CAD build for the part. Positions are in the model's coordinates, mm. Coordinates: 2 decimals unless noted, no trailing zeros. Loops run counter-clockwise (first coordinate to the right, second up) from the corner with the lowest first, then second, coordinate; pieces in that order, holes last. Notation, with made-up numbers: (-17.5, 56) -> (-9.5, 56) arc R3 ccw to (-9.5, 60) -> close; hole circle Ø5 at (24, 41.5). An arc over 180 degrees is marked (long way). Return JSON: item names as keys, results as strings. Group by question number.
(1) Probe L1, parallel to X at y = -20, z = 2.05 (3 decimals); L2, parallel to Y at x = -24.5, z = 1.05; L3, parallel to X at y = -9, z = 2.2 (3 decimals). List the from-to ranges inside material, lowest first.
(2) Flat gauge pin, fed straight in: pin 1 Ø12 at (x, y) = (-93.5, -21) entering from +Z. Where does the tip first touch, or does it go through?
(3) Saw through at C-C on z = 0.8. Give the number of separate pieces and of enclosed holes in the cut face, then the cut area to 3 significant figures.
(4) Saw through at B-B on y = -54.5. Write the cut outline in (x, z) (3 decimals).
(5) Saw through at A-A on x = -134.5. Write the cut outline in (y, z), then the cut area to 3 significant figures.
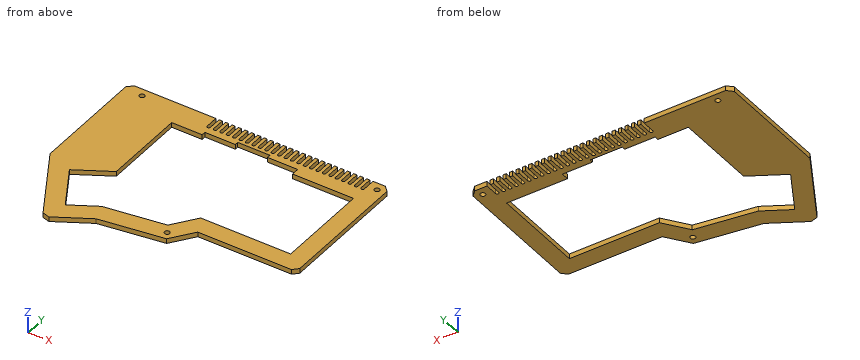
```python
from build123d import *

# Parameters (mm, degrees)
ESQUISSE1_R             = 1.6
BOSS_EXTRU_1_DEPTH      = 3
ENL_V_MAT_EXTRU_1_DEPTH = 10


with BuildPart() as part:
    # Esquisse1 → Boss.-Extru.1 (new body)
    with BuildSketch(Plane.XY):
        Polygon((5.525007543, 0.072428093), (2.276763789, 3.320852512), (-154.236345188, 3.320852512), (-157.478985875, 0.078211825), (-157.478985875, -70.04068474), (-131.779420125, -114.771472067), (-127.355917516, -115.9649154), (-106.081983802, -103.720194839), (-66.092540926, -97.775797545), (-55.98795635, -83.933633781), (2.418252352, -83.933633781), (5.525007543, -80.826878591), align=None)
        Polygon((-126.111124489, -102.556497988), (-140.02282508, -78.342807898), (-141.407217303, -75.981121034), (-120.346626934, -63.796065222), (-120.346308835, -12.429484403), (-101.345774335, -12.429484403), (-101.345774335, -9.929307079), (-82.344426674, -9.929307079), (-82.344426674, -7.679926158), (-62.343149943, -7.681038584), (-62.343149943, -9.929307079), (-43.477687779, -9.929307079), (-43.477687779, -14.679643994), (-5.474992457, -14.679643994), (-5.474992457, -72.933633781), (-61.577157206, -72.933633781), (-72.263087593, -87.572177036), (-109.761976756, -93.1463556), align=None, mode=Mode.SUBTRACT)
        with Locations((-68.897334865, -93.137788223)):
            Circle(ESQUISSE1_R, mode=Mode.SUBTRACT)
        with Locations((-146.02282508, -1.677868186)):
            Circle(ESQUISSE1_R, mode=Mode.SUBTRACT)
        with Locations((0.525007543, -1.68453516)):
            Circle(ESQUISSE1_R, mode=Mode.SUBTRACT)
    extrude(amount=BOSS_EXTRU_1_DEPTH)

    # Esquisse2 → Enlèv. mat.-Extru.1 (cut)
    with BuildSketch(Plane.XY.offset(3)):
        with BuildLine():
            Line((-5.386559375, 6.054162745), (-5.386559375, -4.679147488))
            ThreePointArc((-5.386559375, -4.679147488), (-6.386559375, -5.679147488), (-7.386559375, -4.679147488))
            Line((-7.386559375, -4.679147488), (-7.386559375, 6.054162745))
            ThreePointArc((-7.386559375, 6.054162745), (-6.386559375, 7.054162745), (-5.386559375, 6.054162745))
        make_face()
        with BuildLine():
            Line((-9.386559375, 6.054162745), (-9.386559375, -4.679147488))
            ThreePointArc((-9.386559375, -4.679147488), (-10.386559375, -5.679147488), (-11.386559375, -4.679147488))
            Line((-11.386559375, -4.679147488), (-11.386559375, 6.054162745))
            ThreePointArc((-11.386559375, 6.054162745), (-10.386559375, 7.054162745), (-9.386559375, 6.054162745))
        make_face()
        with BuildLine():
            Line((-13.386559375, 6.054162745), (-13.386559375, -4.679147488))
            ThreePointArc((-13.386559375, -4.679147488), (-14.386559375, -5.679147488), (-15.386559375, -4.679147488))
            Line((-15.386559375, -4.679147488), (-15.386559375, 6.054162745))
            ThreePointArc((-15.386559375, 6.054162745), (-14.386559375, 7.054162745), (-13.386559375, 6.054162745))
        make_face()
        with BuildLine():
            Line((-17.386559375, 6.054162745), (-17.386559375, -4.679147488))
            ThreePointArc((-17.386559375, -4.679147488), (-18.386559375, -5.679147488), (-19.386559375, -4.679147488))
            Line((-19.386559375, -4.679147488), (-19.386559375, 6.054162745))
            ThreePointArc((-19.386559375, 6.054162745), (-18.386559375, 7.054162745), (-17.386559375, 6.054162745))
        make_face()
        with BuildLine():
            Line((-21.386559375, 6.054162745), (-21.386559375, -4.679147488))
            ThreePointArc((-21.386559375, -4.679147488), (-22.386559375, -5.679147488), (-23.386559375, -4.679147488))
            Line((-23.386559375, -4.679147488), (-23.386559375, 6.054162745))
            ThreePointArc((-23.386559375, 6.054162745), (-22.386559375, 7.054162745), (-21.386559375, 6.054162745))
        make_face()
        with BuildLine():
            Line((-25.386559375, 6.054162745), (-25.386559375, -4.679147488))
            ThreePointArc((-25.386559375, -4.679147488), (-26.386559375, -5.679147488), (-27.386559375, -4.679147488))
            Line((-27.386559375, -4.679147488), (-27.386559375, 6.054162745))
            ThreePointArc((-27.386559375, 6.054162745), (-26.386559375, 7.054162745), (-25.386559375, 6.054162745))
        make_face()
        with BuildLine():
            Line((-29.386559375, 6.054162745), (-29.386559375, -4.679147488))
            ThreePointArc((-29.386559375, -4.679147488), (-30.386559375, -5.679147488), (-31.386559375, -4.679147488))
            Line((-31.386559375, -4.679147488), (-31.386559375, 6.054162745))
            ThreePointArc((-31.386559375, 6.054162745), (-30.386559375, 7.054162745), (-29.386559375, 6.054162745))
        make_face()
        with BuildLine():
            Line((-33.386559375, 6.054162745), (-33.386559375, -4.679147488))
            ThreePointArc((-33.386559375, -4.679147488), (-34.386559375, -5.679147488), (-35.386559375, -4.679147488))
            Line((-35.386559375, -4.679147488), (-35.386559375, 6.054162745))
            ThreePointArc((-35.386559375, 6.054162745), (-34.386559375, 7.054162745), (-33.386559375, 6.054162745))
        make_face()
        with BuildLine():
            Line((-37.386559375, 6.054162745), (-37.386559375, -4.679147488))
            ThreePointArc((-37.386559375, -4.679147488), (-38.386559375, -5.679147488), (-39.386559375, -4.679147488))
            Line((-39.386559375, -4.679147488), (-39.386559375, 6.054162745))
            ThreePointArc((-39.386559375, 6.054162745), (-38.386559375, 7.054162745), (-37.386559375, 6.054162745))
        make_face()
        with BuildLine():
            Line((-41.386559375, 6.054162745), (-41.386559375, -4.679147488))
            ThreePointArc((-41.386559375, -4.679147488), (-42.386559375, -5.679147488), (-43.386559375, -4.679147488))
            Line((-43.386559375, -4.679147488), (-43.386559375, 6.054162745))
            ThreePointArc((-43.386559375, 6.054162745), (-42.386559375, 7.054162745), (-41.386559375, 6.054162745))
        make_face()
        with BuildLine():
            Line((-45.386559375, 6.054162745), (-45.386559375, -4.679147488))
            ThreePointArc((-45.386559375, -4.679147488), (-46.386559375, -5.679147488), (-47.386559375, -4.679147488))
            Line((-47.386559375, -4.679147488), (-47.386559375, 6.054162745))
            ThreePointArc((-47.386559375, 6.054162745), (-46.386559375, 7.054162745), (-45.386559375, 6.054162745))
        make_face()
        with BuildLine():
            Line((-49.386559375, 6.054162745), (-49.386559375, -4.679147488))
            ThreePointArc((-49.386559375, -4.679147488), (-50.386559375, -5.679147488), (-51.386559375, -4.679147488))
            Line((-51.386559375, -4.679147488), (-51.386559375, 6.054162745))
            ThreePointArc((-51.386559375, 6.054162745), (-50.386559375, 7.054162745), (-49.386559375, 6.054162745))
        make_face()
        with BuildLine():
            Line((-53.386559375, 6.054162745), (-53.386559375, -4.679147488))
            ThreePointArc((-53.386559375, -4.679147488), (-54.386559375, -5.679147488), (-55.386559375, -4.679147488))
            Line((-55.386559375, -4.679147488), (-55.386559375, 6.054162745))
            ThreePointArc((-55.386559375, 6.054162745), (-54.386559375, 7.054162745), (-53.386559375, 6.054162745))
        make_face()
        with BuildLine():
            Line((-57.386559375, 6.054162745), (-57.386559375, -4.679147488))
            ThreePointArc((-57.386559375, -4.679147488), (-58.386559375, -5.679147488), (-59.386559375, -4.679147488))
            Line((-59.386559375, -4.679147488), (-59.386559375, 6.054162745))
            ThreePointArc((-59.386559375, 6.054162745), (-58.386559375, 7.054162745), (-57.386559375, 6.054162745))
        make_face()
        with BuildLine():
            Line((-61.386559375, 6.054162745), (-61.386559375, -4.679147488))
            ThreePointArc((-61.386559375, -4.679147488), (-62.386559375, -5.679147488), (-63.386559375, -4.679147488))
            Line((-63.386559375, -4.679147488), (-63.386559375, 6.054162745))
            ThreePointArc((-63.386559375, 6.054162745), (-62.386559375, 7.054162745), (-61.386559375, 6.054162745))
        make_face()
        with BuildLine():
            Line((-65.386559375, 6.054162745), (-65.386559375, -4.679147488))
            ThreePointArc((-65.386559375, -4.679147488), (-66.386559375, -5.679147488), (-67.386559375, -4.679147488))
            Line((-67.386559375, -4.679147488), (-67.386559375, 6.054162745))
            ThreePointArc((-67.386559375, 6.054162745), (-66.386559375, 7.054162745), (-65.386559375, 6.054162745))
        make_face()
        with BuildLine():
            Line((-69.386559375, 6.054162745), (-69.386559375, -4.679147488))
            ThreePointArc((-69.386559375, -4.679147488), (-70.386559375, -5.679147488), (-71.386559375, -4.679147488))
            Line((-71.386559375, -4.679147488), (-71.386559375, 6.054162745))
            ThreePointArc((-71.386559375, 6.054162745), (-70.386559375, 7.054162745), (-69.386559375, 6.054162745))
        make_face()
        with BuildLine():
            Line((-73.386559375, 6.054162745), (-73.386559375, -4.679147488))
            ThreePointArc((-73.386559375, -4.679147488), (-74.386559375, -5.679147488), (-75.386559375, -4.679147488))
            Line((-75.386559375, -4.679147488), (-75.386559375, 6.054162745))
            ThreePointArc((-75.386559375, 6.054162745), (-74.386559375, 7.054162745), (-73.386559375, 6.054162745))
        make_face()
        with BuildLine():
            Line((-77.386559375, 6.054162745), (-77.386559375, -4.679147488))
            ThreePointArc((-77.386559375, -4.679147488), (-78.386559375, -5.679147488), (-79.386559375, -4.679147488))
            Line((-79.386559375, -4.679147488), (-79.386559375, 6.054162745))
            ThreePointArc((-79.386559375, 6.054162745), (-78.386559375, 7.054162745), (-77.386559375, 6.054162745))
        make_face()
        with BuildLine():
            Line((-81.386559375, 6.054162745), (-81.386559375, -4.679147488))
            ThreePointArc((-81.386559375, -4.679147488), (-82.386559375, -5.679147488), (-83.386559375, -4.679147488))
            Line((-83.386559375, -4.679147488), (-83.386559375, 6.054162745))
            ThreePointArc((-83.386559375, 6.054162745), (-82.386559375, 7.054162745), (-81.386559375, 6.054162745))
        make_face()
        with BuildLine():
            Line((-85.386559375, 6.054162745), (-85.386559375, -4.679147488))
            ThreePointArc((-85.386559375, -4.679147488), (-86.386559375, -5.679147488), (-87.386559375, -4.679147488))
            Line((-87.386559375, -4.679147488), (-87.386559375, 6.054162745))
            ThreePointArc((-87.386559375, 6.054162745), (-86.386559375, 7.054162745), (-85.386559375, 6.054162745))
        make_face()
        with BuildLine():
            Line((-89.386559375, 6.054162745), (-89.386559375, -4.679147488))
            ThreePointArc((-89.386559375, -4.679147488), (-90.386559375, -5.679147488), (-91.386559375, -4.679147488))
            Line((-91.386559375, -4.679147488), (-91.386559375, 6.054162745))
            ThreePointArc((-91.386559375, 6.054162745), (-90.386559375, 7.054162745), (-89.386559375, 6.054162745))
        make_face()
        with BuildLine():
            Line((-93.386559375, 6.054162745), (-93.386559375, -4.679147488))
            ThreePointArc((-93.386559375, -4.679147488), (-94.386559375, -5.679147488), (-95.386559375, -4.679147488))
            Line((-95.386559375, -4.679147488), (-95.386559375, 6.054162745))
            ThreePointArc((-95.386559375, 6.054162745), (-94.386559375, 7.054162745), (-93.386559375, 6.054162745))
        make_face()
        with BuildLine():
            Line((-97.386559375, 6.054162745), (-97.386559375, -4.679147488))
            ThreePointArc((-97.386559375, -4.679147488), (-98.386559375, -5.679147488), (-99.386559375, -4.679147488))
            Line((-99.386559375, -4.679147488), (-99.386559375, 6.054162745))
            ThreePointArc((-99.386559375, 6.054162745), (-98.386559375, 7.054162745), (-97.386559375, 6.054162745))
        make_face()
        with BuildLine():
            Line((-101.386559375, 6.054162745), (-101.386559375, -4.679147488))
            ThreePointArc((-101.386559375, -4.679147488), (-102.386559375, -5.679147488), (-103.386559375, -4.679147488))
            Line((-103.386559375, -4.679147488), (-103.386559375, 6.054162745))
            ThreePointArc((-103.386559375, 6.054162745), (-102.386559375, 7.054162745), (-101.386559375, 6.054162745))
        make_face()
    extrude(amount=-ENL_V_MAT_EXTRU_1_DEPTH, mode=Mode.SUBTRACT)


solid = part.part
```
Geometry results:
{
 "1": {"L1": "-157.479 to -120.346, -5.475 to 5.525", "L2": "-83.93 to -72.93, -14.68 to 3.32", "L3": "-157.479 to -82.344, -62.343 to 5.525"},
 "2": {"pin 1": "through"},
 "3": {"separate pieces": "1", "enclosed holes": "4", "area": "6,890 mm²"},
 "4": {"outline": "(-157.479, 0) -> (-120.347, 0) -> (-120.347, 3) -> (-157.479, 3) -> close; (-5.475, 0) -> (5.525, 0) -> (5.525, 3) -> (-5.475, 3) -> close"},
 "5": {"outline": "(-110.04, 0) -> (-87.96, 0) -> (-87.96, 3) -> (-110.04, 3) -> close; (-71.98, 0) -> (3.32, 0) -> (3.32, 3) -> (-71.98, 3) -> close", "area": "292 mm²"}
}
